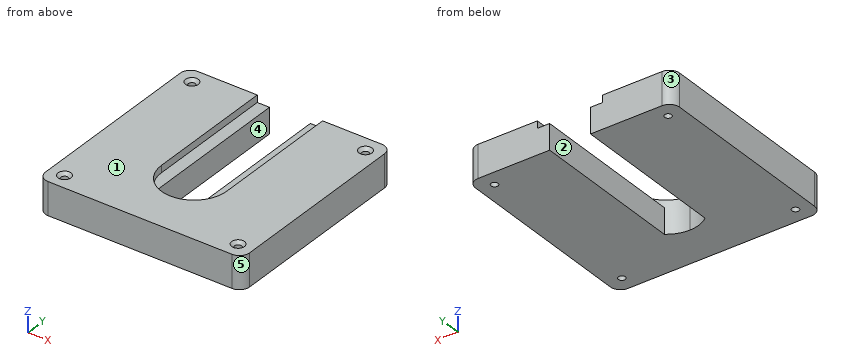
from build123d import *

# Parameters (mm, degrees)
SKETCH1_W                                    = 100
SKETCH1_H                                    = 100
BOSS_EXTRUDE1_DEPTH                          = 16
SKETCH2_W                                    = 100
SKETCH2_H                                    = 100
BOSS_EXTRUDE2_DEPTH                          = 16
CUT_EXTRUDE1_DEPTH                           = 80
BOSS_EXTRUDE3_DEPTH                          = 16
BOSS_EXTRUDE4_REACH                          = 75.763
CSK_FOR_M3_COUNTERSUNK_FLAT_HEAD_SCR_2_COUNT = 2
CSK_FOR_M3_COUNTERSUNK_FLAT_HEAD_SCR_2_PITCH = 85
CSK_FOR_M3_COUNTERSUNK_FLAT_HEAD_SCR_3_COUNT = 2
CSK_FOR_M3_COUNTERSUNK_FLAT_HEAD_SCR_3_PITCH = 120.208152802
CSK_FOR_M3_COUNTERSUNK_FLAT_HEAD_SCR_4_COUNT = 2
CSK_FOR_M3_COUNTERSUNK_FLAT_HEAD_SCR_4_PITCH = 85
FILLET1_R                                    = 5
FILLET2_R                                    = 5


with BuildPart() as part:
    # Sketch1 → Boss-Extrude1 (new body)
    with BuildSketch(Plane.XY):
        Rectangle(SKETCH1_W, SKETCH1_H)
    extrude(amount=BOSS_EXTRUDE1_DEPTH)


with BuildPart() as body_2:
    # Sketch2 → Boss-Extrude2 (new body)
    with BuildSketch(Plane.XY.offset(16)):
        Rectangle(SKETCH2_W, SKETCH2_H)
    extrude(amount=BOSS_EXTRUDE2_DEPTH)


with BuildPart() as cut_extrude1_tool:
    # Sketch3 → Cut-Extrude1 (new body)
    with BuildSketch(Plane(origin=(0, 50, 0), x_dir=(1, 0, 0), z_dir=(0, 1, 0))):
        Polygon((-16, -32), (-16, -28.5), (-10, -28.5), (-10, -16), (-16, -16), (-16, -11), (16, -11), (16, -16), (10, -16), (10, -28.5), (16, -28.5), (16, -32), align=None)
    extrude(amount=-CUT_EXTRUDE1_DEPTH)


with BuildPart() as part_1:
    add(part.part)

    # Cut-Extrude1: cut by cut_extrude1_tool
    add(cut_extrude1_tool.part, mode=Mode.SUBTRACT)



with BuildPart() as body_2_1:
    add(body_2.part)

    # Cut-Extrude1: cut by cut_extrude1_tool
    add(cut_extrude1_tool.part, mode=Mode.SUBTRACT)

    # Sketch4 → Boss-Extrude3 (add)
    with BuildSketch(Plane.XY.offset(32)):
        with BuildLine():
            Line((-16, -14), (-16, -30))
            Line((-16, -30), (0, -30))
            ThreePointArc((0, -30), (-11.313708499, -25.313708499), (-16, -14))
        make_face()
        with BuildLine():
            ThreePointArc((16, -14), (11.313708499, -25.313708499), (0, -30))
            Line((0, -30), (16, -30))
            Line((16, -30), (16, -14))
        make_face()
    extrude(amount=-BOSS_EXTRUDE3_DEPTH)


with BuildPart() as part_2:
    add(part_1.part)

    # Sketch5 → Boss-Extrude4 (add, up to next)
    with BuildSketch(Plane.XY.offset(11), mode=Mode.PRIVATE) as boss_extrude4_sk1:
        with BuildLine():
            Line((16, -30), (16, -14))
            ThreePointArc((16, -14), (11.313708487, -25.313708511), (-3.4e-08, -30))
            Line((-3.4e-08, -30), (16, -30))
        make_face()
    boss_extrude4_tool1 = extrude(boss_extrude4_sk1.sketch, amount=BOSS_EXTRUDE4_REACH, mode=Mode.PRIVATE) - body_2_1.part
    # Sketch5 → Boss-Extrude4 (add, up to next)
    with BuildSketch(Plane.XY.offset(11), mode=Mode.PRIVATE) as boss_extrude4_sk2:
        with BuildLine():
            ThreePointArc((-3.4e-08, -30), (-11.313708511, -25.313708487), (-16, -14))
            Line((-16, -14), (-16, -30))
            Line((-16, -30), (-3.4e-08, -30))
        make_face()
    boss_extrude4_tool2 = extrude(boss_extrude4_sk2.sketch, amount=BOSS_EXTRUDE4_REACH, mode=Mode.PRIVATE) - body_2_1.part
    add(boss_extrude4_tool1.solids().sort_by_distance((12.426113, -26.426113, 11))[0])
    add(boss_extrude4_tool2.solids().sort_by_distance((-12.426113, -26.426113, 11))[0])


with BuildPart() as csk_for_m3_countersunk_flat_head_screw1_tool:
    # Sketch7 → CSK for M3 Countersunk Flat Head Screw1 (revolve)
    with BuildSketch(Plane(origin=(-42.5, 42.5, 32), x_dir=(0, -1, 0), z_dir=(1, 0, 0))):
        Polygon((0, 0), (0, 32), (1.7, 32), (1.7, 1.45), (3.15, 0), align=None)
    csk_for_m3_countersunk_flat_head_screw1 = revolve(axis=Axis((-42.5, 42.5, 38.35), (0, 0, -1)))


with BuildPart() as part_3:
    add(part_2.part)

    # CSK for M3 Countersunk Flat Head Screw1: cut by csk_for_m3_countersunk_flat_head_screw1_tool
    add(csk_for_m3_countersunk_flat_head_screw1_tool.part, mode=Mode.SUBTRACT)


with BuildPart() as body_2_2:
    add(body_2_1.part)

    # CSK for M3 Countersunk Flat Head Screw1: cut by csk_for_m3_countersunk_flat_head_screw1_tool
    add(csk_for_m3_countersunk_flat_head_screw1_tool.part, mode=Mode.SUBTRACT)


with BuildPart() as csk_for_m3_countersunk_flat_head_scr_2_tool:
    # CSK for M3 Countersunk Flat Head Scr 2: CSK for M3 Countersunk Flat Head Screw1 ×2
    with Locations(*[(i * CSK_FOR_M3_COUNTERSUNK_FLAT_HEAD_SCR_2_PITCH, 0, 0) for i in range(1, CSK_FOR_M3_COUNTERSUNK_FLAT_HEAD_SCR_2_COUNT)]):
        add(csk_for_m3_countersunk_flat_head_screw1)


with BuildPart() as part_4:
    add(part_3.part)

    # CSK for M3 Countersunk Flat Head Scr 2: cut by csk_for_m3_countersunk_flat_head_scr_2_tool
    add(csk_for_m3_countersunk_flat_head_scr_2_tool.part, mode=Mode.SUBTRACT)


with BuildPart() as body_2_3:
    add(body_2_2.part)

    # CSK for M3 Countersunk Flat Head Scr 2: cut by csk_for_m3_countersunk_flat_head_scr_2_tool
    add(csk_for_m3_countersunk_flat_head_scr_2_tool.part, mode=Mode.SUBTRACT)


with BuildPart() as csk_for_m3_countersunk_flat_head_scr_3_tool:
    # CSK for M3 Countersunk Flat Head Scr 3: CSK for M3 Countersunk Flat Head Screw1 ×2
    with Locations(*[Vector(0.7071067811865476, -0.7071067811865476, 0) * (i * CSK_FOR_M3_COUNTERSUNK_FLAT_HEAD_SCR_3_PITCH) for i in range(1, CSK_FOR_M3_COUNTERSUNK_FLAT_HEAD_SCR_3_COUNT)]):
        add(csk_for_m3_countersunk_flat_head_screw1)


with BuildPart() as part_5:
    add(part_4.part)

    # CSK for M3 Countersunk Flat Head Scr 3: cut by csk_for_m3_countersunk_flat_head_scr_3_tool
    add(csk_for_m3_countersunk_flat_head_scr_3_tool.part, mode=Mode.SUBTRACT)


with BuildPart() as body_2_4:
    add(body_2_3.part)

    # CSK for M3 Countersunk Flat Head Scr 3: cut by csk_for_m3_countersunk_flat_head_scr_3_tool
    add(csk_for_m3_countersunk_flat_head_scr_3_tool.part, mode=Mode.SUBTRACT)


with BuildPart() as csk_for_m3_countersunk_flat_head_scr_4_tool:
    # CSK for M3 Countersunk Flat Head Scr 4: CSK for M3 Countersunk Flat Head Screw1 ×2
    with Locations(*[(0, -i * CSK_FOR_M3_COUNTERSUNK_FLAT_HEAD_SCR_4_PITCH, 0) for i in range(1, CSK_FOR_M3_COUNTERSUNK_FLAT_HEAD_SCR_4_COUNT)]):
        add(csk_for_m3_countersunk_flat_head_screw1)


with BuildPart() as part_6:
    add(part_5.part)

    # CSK for M3 Countersunk Flat Head Scr 4: cut by csk_for_m3_countersunk_flat_head_scr_4_tool
    add(csk_for_m3_countersunk_flat_head_scr_4_tool.part, mode=Mode.SUBTRACT)

    # Fillet2
    fillet2_edges = [part_6.edges().sort_by_distance(p)[0] for p in [
        (-50, -50, 8),
        (-50, 50, 8),
        (50, 50, 8),
        (50, -50, 8),
    ]]
    fillet(fillet2_edges, radius=FILLET2_R)


with BuildPart() as body_2_5:
    add(body_2_4.part)

    # CSK for M3 Countersunk Flat Head Scr 4: cut by csk_for_m3_countersunk_flat_head_scr_4_tool
    add(csk_for_m3_countersunk_flat_head_scr_4_tool.part, mode=Mode.SUBTRACT)

    # Fillet1
    fillet1_edges = [body_2_5.edges().sort_by_distance(p)[0] for p in [
        (-50, 50, 24),
        (50, 50, 24),
        (50, -50, 24),
        (-50, -50, 24),
    ]]
    fillet(fillet1_edges, radius=FILLET1_R)


solid = body_2_5.part
Part model, mm, in its own coordinate system. Face numbers are marked on the shaded views. A direction names the side the tool comes from. Give positions to 0.01 mm unless a question says otherwise; leave off trailing zeros. Write each loop counter-clockwise with the first axis right and the second up, starting at its lowest first coordinate (ties: lowest second). Pieces come first, ordered by that corner, then holes.
1) Pin check, flat tips, straight feed: pin 1 (1.8 mm diameter, centred on x = -13, y = -6.5, fed in from +Z); pin 2 (1 mm diameter, centred on x = -2, z = 27, fed in from +Y); pin 3 (5.5 mm diameter, centred on x = -42.5, y = -42.5, fed in from +Z). Stop position of each tip, or through.
Resolved:
pin 1: stops at z = 28.5
pin 2: stops at y = -29.8
pin 3: stops at z = 31.6
2) Cut at B-B on z = 21.25. Write the cut outline in (x, y), then the cut area to 3 significant figures.
Resolved:
outline: (-50, -45) arc R5 ccw to (-45, -50) - (45, -50) arc R5 ccw to (50, -45) - (50, 45) arc R5 ccw to (45, 50) - (10, 50) - (10, -26.49) arc R16 cw to (-10, -26.49) - (-10, 50) - (-45, 50) arc R5 ccw to (-50, 45) - close; hole circle Ø3.4 at (-42.5, -42.5); hole circle Ø3.4 at (-42.5, 42.5); hole circle Ø3.4 at (42.5, -42.5); hole circle Ø3.4 at (42.5, 42.5)
area: 8,360 mm2
3) Cut at A-A on y = -42.5. Write the cut outline in (x, z).
Resolved:
outline: (-50, 16) - (-44.2, 16) - (-44.2, 30.55) - (-45.65, 32) - (-50, 32) - close; (-40.8, 16) - (40.8, 16) - (40.8, 30.55) - (39.35, 32) - (-39.35, 32) - (-40.8, 30.55) - close; (44.2, 16) - (50, 16) - (50, 32) - (45.65, 32) - (44.2, 30.55) - close
4) Two-plate mould, pull along X, no slides. Class the marked faces 3, 4 and 5: released by +X, released by -X, zero draft, split by the parting line, or undercut.
Resolved:
face 3: released by -X
face 4: undercut
face 5: released by +X
5) Probe L1, parallel to X at y = 42.5, z = 25.25; L2, parallel to Y at x = -42.5, z = 23.75; L3, parallel to X at y = -12, z = 19.5. List the from-to ranges inside material, lowest first.
Resolved:
L1: x = -50 to -44.2, -40.8 to -10, 10 to 40.8, 44.2 to 50
L2: y = -50 to -44.2, -40.8 to 40.8, 44.2 to 50
L3: x = -50 to -10, 10 to 50
6) Cut at D-D on y = -12. Write the cut outline in (x, z).
Resolved:
outline: (-50, 16) - (-10, 16) - (-10, 28.5) - (-16, 28.5) - (-16, 32) - (-50, 32) - close; (10, 16) - (50, 16) - (50, 32) - (16, 32) - (16, 28.5) - (10, 28.5) - close
7) Which spindle directions (+Z, -Z, +X, -X, +Y, -Y) get a long thin tool onto all of the face, cutting with end or side? Do the marked faces 1 and 2. Say none if no direction does.
Resolved:
face 1: +Z, +X, -X, +Y, -Y
face 2: +Z, -Z, +Y
